Design review of the part built by this model. Coordinates are the model's own, in mm. A direction names the side the tool comes from. Coordinates: 2 decimals unless noted, no trailing zeros. Write each loop counter-clockwise with the first axis right and the second up, starting at its lowest first coordinate (ties: lowest second). Pieces come first, ordered by that corner, then holes. Notation, with made-up numbers: M -28,44 L 3,44 A9 cw 3,58 Z; hole C 71.5,-34.5 d10. An arc over 180 degrees is marked long. One line per question, with ' | ' between items.
from build123d import *

# Parameters (mm, degrees)
F0_R     = 36.211569
F1_DEPTH = 7


with BuildPart() as f1:
    # F0 (on Top) → F1 (new body)
    with BuildSketch(Plane.XY):
        with Locations((2.013676, 0)):
            Circle(F0_R)
        Polygon((3.347939, -24.192038), (-14.739004, -19.473705), (-24.192038, -3.347939), (-19.473705, 14.739004), (-3.347939, 24.192038), (14.739004, 19.473705), (24.192038, 3.347939), (19.473705, -14.739004), align=None, mode=Mode.SUBTRACT)
    extrude(amount=F1_DEPTH)


solid = f1.part
1. To check wall thickness, follow line 1 along Y through (x, z) = (5, 1); line 2 along Y through (x, z) = (17, 4.5); line 3 along X through (y, z) = (7.5, 6.75). State the ranges of each line that lie inside material, in increasing order. Write a range as [from, to].
Answer sheet:
line 1: [-36.09, -23.22], [22.01, 36.09] | line 2: [-32.96, -16.19], [15.62, 32.96] | line 3: [-33.41, -21.36], [21.76, 37.44]
2. Tool access review of faces 4 (the face through (19.4, 11.52, 3.45)), 5 (the face through (18, 17, 7)): name each direction out of +Z, -Z, +X, -X, +Y, -Y from which nothing blocks a thin tool from reaching the whole face with its end or side.
Answer sheet:
face 4: +Z, -Z | face 5: +Z, +X, -X, +Y, -Y
3. Take a section at B-B (x = -1). Write out the cut boundary in (y, z).
Answer sheet:
outline: M -36.09,0 L -23.06,0 L -23.06,7 L -36.09,7 Z; M 23.58,0 L 36.09,0 L 36.09,7 L 23.58,7 Z
4. Draft analysis for pull direction Y (two halves, no side actions). For faces 1 (the face through (18, 17, 0)), 2 (the face through (36.553, 10.877, 3.451)), 3 (the face through (-11.52, 19.4, 3.45)), state which applies: pulls with the +Y half, pulls with the -Y half, needs draft (parallel to the pull), parting line crosses it, or undercut.
Answer sheet:
face 1: needs draft | face 2: parting line crosses it | face 3: undercut
5. Insertion check: pin 1 Ø1 at (y, z) = (18.5, 3.5) entering from -X; pin 2 Ø4 at (y, z) = (26, 1) entering from +X; pin 3 Ø4 at (x, z) = (7, 3) entering from +Y. Each pin has a flat end and moves straight along its axis. Give the tip position at first contact, or say it passes through.
Answer sheet:
pin 1: x = -29.41 | pin 2: x = 29.13 | pin 3: y = 36.09
6. Take a section at A-A (y = -6.5). Write out the cut boundary in (x, z).
Answer sheet:
outline: M -33.61,0 L -22.34,0 L -22.34,7 L -33.61,7 Z; M 21.62,0 L 37.64,0 L 37.64,7 L 21.62,7 Z
7. Take a section at C-C (z = 4.5). Write out the cut boundary in (x, y), then the cut area to 3 significant figures.
Answer sheet:
outline: C 2.01,0 d72.42; hole M -24.19,-3.35 L -14.74,-19.47 L 3.35,-24.19 L 19.47,-14.74 L 24.19,3.35 L 14.74,19.47 L -3.35,24.19 L -19.47,14.74 Z | area: 2,430 mm^2
